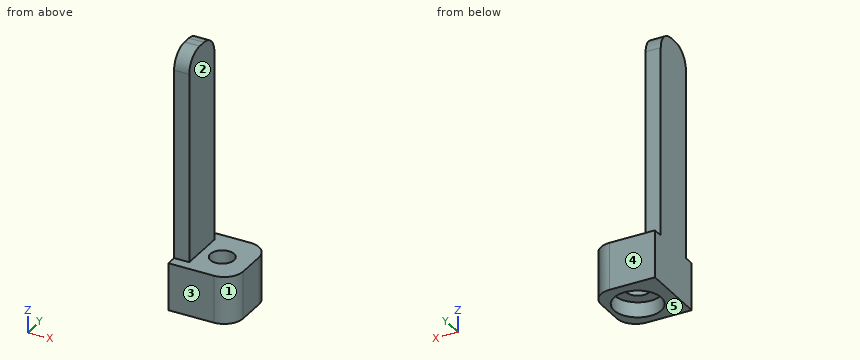
```python
from build123d import *

# Parameters (mm, degrees)
F1_DEPTH  = 5
F2_R      = 2.5
F3_DEPTH  = 1.6
F4_R      = 1.25
F5_DEPTH  = 3.4
F6_W      = 2
F6_H      = 4.8
F7_DEPTH  = 22
F8_R      = 2
F9_DEPTH  = 0.2
F10_DEPTH = 0.2


# Not quite as in the source:
# - a feature names something its author has since deleted; it is built from what else it names


with BuildPart() as f1:
    # F0 (on Top) → F1 (new body)
    with BuildSketch(Plane.XY):
        with BuildLine():
            Line((1, 21.8148477226), (-4, 21.8148477226))
            Line((-4, 21.8148477226), (-4, 14.8148477226))
            Line((-4, 14.8148477226), (1, 14.8148477226))
            ThreePointArc((1, 14.8148477226), (2.4142135624, 15.4006341603), (3, 16.8148477226))
            Line((3, 16.8148477226), (3, 19.8148477226))
            ThreePointArc((3, 19.8148477226), (2.4142135624, 21.229061285), (1, 21.8148477226))
        make_face()
    extrude(amount=F1_DEPTH)

    # F2 (on face) → F3 (cut)
    with BuildSketch(Plane(origin=(0, 0, 0), x_dir=(1, 0, 0), z_dir=(0, 0, -1))):
        with Locations((0, -18.2346012443)):
            Circle(F2_R)
    extrude(amount=-F3_DEPTH, mode=Mode.SUBTRACT)

    # F4 (on face) → F5 (cut)
    with BuildSketch(Plane(origin=(0, 0, 1.6), x_dir=(1, 0, 0), z_dir=(0, 0, -1))):
        with Locations((0, -18.2346012443)):
            Circle(F4_R)
    extrude(amount=-F5_DEPTH, mode=Mode.SUBTRACT)

    # F6 (on face) → F7 (join)
    with BuildSketch(Plane.XY.offset(5)):
        with Locations((-3, 18.3148477226)):
            Rectangle(F6_W, F6_H)
    extrude(amount=F7_DEPTH)

    # F8
    f8_edges = [f1.edges().sort_by_distance(p)[0] for p in [
        (-3, 20.714848, 27),
        (-3, 15.914848, 27),
    ]]
    fillet(f8_edges, radius=F8_R)

    # F9 (cut): a face of the model
    f9_faces = [f1.faces().sort_by_distance(p)[0] for p in [
        (-2, 18.3148477226, 15.8255925745),
    ]]
    extrude(f9_faces, amount=-F9_DEPTH, mode=Mode.SUBTRACT)

    # F10 (cut): a face of the model
    f10_faces = [f1.faces().sort_by_distance(p)[0] for p in [
        (-4, 18.3148477226, 12.4674053391),
    ]]
    extrude(f10_faces, amount=-F10_DEPTH, mode=Mode.SUBTRACT)


solid = f1.part
```
CAD build for the part. Positions are in the model's coordinates, mm. Face numbers are marked on the shaded views. A direction names the side the tool comes from. Coordinates: 2 decimals unless noted, no trailing zeros. Order: outer loops, then holes, each group sorted by start corner. A loop starts at its lowest first (then second) coordinate and runs counter-clockwise, first axis right, second up. Notation, with made-up numbers: M -35.75,41.25 L -9.75,41.25 A25 cw -9.75,64.25 Z; hole C 65,46 d3. An arc over 180 degrees is marked long. Write each question's results on one line, items separated by ' | '. Start each with the question number.
Q1. Cut at C-C (z = 3.5). List the corners of the cut face in (x, y).
Q2. Cut at B-B (y = 19). List the corners of the cut face in (x, z).
Q3. Flat gauge pins, fed straight in: P1, Ø1.8, axis at x = -3, z = 11, coming from the -Y side; P2, Ø1, axis at x = -0.5, z = 6, coming from the +Y side; P3, Ø1.4, axis at y = 18.5, z = 16, coming from the +X side; P4, Ø0.5, axis at x = -3, z = 13, coming from the +Y side. Where does each tip first touch, or does it go through?
Q4. Cut at A-A (x = 0). List the corners of the cut face in (y, z), then the cut area to 3 significant figures.
Q5. Pull direction Y, two halves, no side cores. Call the marked faces 3, 4 and 5: +Y half, -Y half, draft (parallel to the pull), parting line (faces both ways), or undercut.
Q6. Cut at D-D (z = 13.25). List the corners of the cut face in (x, y), then the cut area to 3 significant figures.
Q7. Drill centre lines: probe 1 along Y at (x, z) = (0, 1.2); probe 2 along Y at (x, z) = (0, 2.8); probe 3 along Y at (x, z) = (-2.5, 8.5). Where is each one in solid material? Low to high. Write a range as from..to.
Q8. Which spindle directions (+Z, -Z, +X, -X, +Y, -Y) get a long thin tool onto all of the face, cutting with end or side? Do the marked faces 1 and 2. Say none if no direction does.
Found:
1) outline: M -3.8,14.81 L 1,14.81 A2 ccw 3,16.81 L 3,19.81 A2 ccw 1,21.81 L -3.8,21.81 Z; hole C 0,18.23 d2.5
2) outline: M -3.8,0 L -2.38,0 L -2.38,1.6 L -0.99,1.6 L -0.99,5 L -2.2,5 L -2.2,26.98 L -3.8,26.98 Z; M 0.99,1.6 L 2.38,1.6 L 2.38,0 L 3,0 L 3,5 L 0.99,5 Z
3) P1: y = 15.91 | P2: through | P3: x = -2.2 | P4: y = 20.71
4) outline: M 14.81,0 L 15.73,0 L 15.73,1.6 L 16.98,1.6 L 16.98,5 L 14.81,5 Z; M 19.48,1.6 L 20.73,1.6 L 20.73,0 L 21.81,0 L 21.81,5 L 19.48,5 Z | area: 18.5 mm²
5) face 3: -Y half | face 4: +Y half | face 5: draft
6) outline: M -3.8,15.91 L -2.2,15.91 L -2.2,20.71 L -3.8,20.71 Z | area: 7.68 mm²
7) probe 1: 14.81..15.73, 20.73..21.81 | probe 2: 14.81..16.98, 19.48..21.81 | probe 3: 15.91..20.71
8) face 1: +Z, -Z, +X, -Y | face 2: +Z, +X, +Y, -Y
